Check sheet for the modelled part. Datum: model origin and axes. Units: mm. Round coordinates to 2 decimals unless told otherwise and drop trailing zeros. Write each loop counter-clockwise with the first axis right and the second up, starting at its lowest first coordinate (ties: lowest second). Pieces come first, ordered by that corner, then holes. Notation, with made-up numbers: (50.5, 1) - (96.5, 1) arc R24 ccw to (96.5, 34) - close; hole circle Ø10 at (56.25, 44). An arc over 180 degrees is marked (long way). Use one line per item in the form item = value. Start each with the question number.
1) Draft check along X on faces 1 (the face through (0, 10, 1)), 2 (the face through (22.944, 0, 1)), 3 (the face through (-17.24, -3.33, 1.52)). Enter one of: +X half, -X half, draft (parallel to the pull), parting line (faces both ways), or undercut.
2) Section check A-A (x = -15). Record the boundary of the cut face in (y, z).
3) Scan lines: probe 1 along X at (y, z) = (-0.75, 1.05); probe 2 along X at (y, z) = (-2.5, 1.1). Record each from-to range of solid material in increasing order.
4) Gauge pin test, flat end, axial feed: P1, Ø5, axis at x = 6.5, y = -8, coming from the -Z side. Record the tip position at first contact, or that the pin passes through.
from build123d import *

# Parameters (mm, degrees)
F0_W          = 45.8885646038
F0_H          = 20
F1_DEPTH      = 3
F2_R          = 2
F3_DEPTH      = 52
F3_DEPTH_BACK = 25


# Not quite as in the source:
# - an extrude ends at something that could not be found from the text; its depth is read off the source's solid


with BuildPart() as f1:
    # F0 (on Top) → F1 (new body)
    with BuildSketch(Plane.XY):
        Rectangle(F0_W, F0_H)
    extrude(amount=F1_DEPTH)

    # F2 (on face) → F3 (cut, two sides)
    with BuildSketch(Plane.XY.offset(3)) as f3_sk:
        with Locations((-15.6491361558, -2.1147204097)):
            Circle(F2_R)
    extrude(amount=F3_DEPTH, mode=Mode.SUBTRACT)
    extrude(f3_sk.sketch, amount=-F3_DEPTH_BACK, mode=Mode.SUBTRACT)


solid = f1.part
Results are:
q1.face_1 = draft
q1.face_2 = +X half
q1.face_3 = undercut
q2.outline = (-10, 0) - (-4.01, 0) - (-4.01, 3) - (-10, 3) - close; (-0.22, 0) - (10, 0) - (10, 3) - (-0.22, 3) - close
q3.probe_1 = -22.94 to -17.11, -14.19 to 22.94
q3.probe_2 = -22.94 to -17.61, -13.69 to 22.94
q4.P1 = 0
